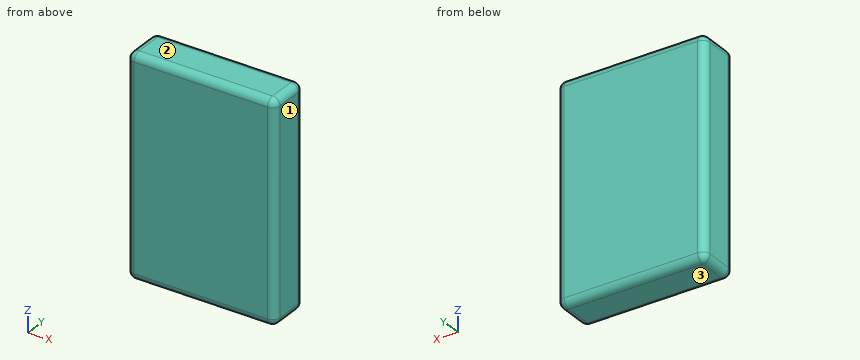
Autodesk Inventor part; units mm, degrees
ref_plane "YZ Plane" through (0, 0, 0) normal (1, 0, 0) x (0, 1, 0)
ref_plane "XZ Plane" through (0, 0, 0) normal (0, 1, 0) x (-1, 0, 0)
ref_plane "XY Plane" through (0, 0, 0) normal (0, 0, 1) x (1, 0, 0)
sketch "Sketch1" plane through (0, 0, 0) normal (0, 1, 0) x (-1, 0, 0)
  line L0 (-32.004, 46.99) -> (32.004, 46.99)
  line L1 (32.004, 46.99) -> (32.004, -46.99)
  line L2 (32.004, -46.99) -> (-32.004, -46.99)
  line L3 (-32.004, -46.99) -> (-32.004, 46.99)
  line L4 (-32.004, 46.99) -> (32.004, -46.99) construction
  line L5 (32.004, 46.99) -> (-32.004, -46.99) construction
  point P0 (0, 0)
  dimension "d0" = 64.008
  dimension "d1" = 93.98
extrude "Extrusion1" add sketch "Sketch1" along normal mid plane 18.034
fillet "Fillet1" radius 3.175 12 edges at (32.004, 9.017, 0) (32.004, -9.017, 0) (32.004, 0, 46.99) (-32.004, 9.017, 0) (0, 9.017, 46.99) (-32.004, 0, 46.99) (0, -9.017, 46.99) (-32.004, -9.017, 0) (-32.004, 0, -46.99) (0, 9.017, -46.99) (0, -9.017, -46.99) (32.004, 0, -46.99)
properties part number "ColdBye_Battery"
The listing builds one solid part. Answer for the finished solid, in the listing's coordinates (mm). Face numbers are marked on the shaded views. Give positions to 0.01 mm unless a question says otherwise; leave off trailing zeros. Order: outer loops, then holes, each group sorted by start corner. A loop starts at its lowest first (then second) coordinate and runs counter-clockwise, first axis right, second up. Notation, with made-up numbers: M 54,86.5 L 59,86.5 A35 cw 59,124.5 Z; hole C 40.25,59.5 d7. An arc over 180 degrees is marked long. Put each result on its own line as item: value. Start each with the question number.
Item 1: The part is cut by section A-A, the plane y = 7.5. Determine the outline of the cut face in (x, z) (3 decimals).
Item 2: For a pull along Z with two mould halves and no side action, classify the marked faces 1, 2 and 3 as +Z half, -Z half, draft (parallel to the pull), parting line (faces both ways), or undercut.
Item 3: Find the intervals of material crossed by line 1 along X through (y, z) = (-6, 3.5); line 2 along X through (y, z) = (-7, -35.5); line 3 along Z through (x, y) = (-24.5, 7.5), in increasing order.
Answer key:
1. outline: M -31.537,-43.815 A2.708 ccw -28.829,-46.523 L 28.829,-46.523 A2.708 ccw 31.537,-43.815 L 31.537,43.815 A2.708 ccw 28.829,46.523 L -28.829,46.523 A2.708 ccw -31.537,43.815 Z
2. face 1: draft
2. face 2: +Z half
2. face 3: -Z half
3. line 1: x = -32 to 32
3. line 2: x = -31.79 to 31.79
3. line 3: z = -46.52 to 46.52
